from build123d import *

# Parameters (mm, degrees)
F1_DEPTH = 10
F3_DEPTH = 4.4
F4_R     = 7.5
F5_DEPTH = 3
F6_R     = 3
F7_DEPTH = 13.001


with BuildPart() as f1:
    # F0 (on Top) → F1 (new body)
    with BuildSketch(Plane.XY):
        with BuildLine():
            ThreePointArc((5.928073, 14.86129), (0, 19.582365), (-5.928073, 14.86129))
            ThreePointArc((-5.928073, 14.86129), (-6.94214, 14.415502), (-7.922931, 13.900617))
            ThreePointArc((-7.922931, 13.900617), (-15.31011, 12.209405), (-15.315118, 4.631108))
            ThreePointArc((-15.315118, 4.631108), (-15.598847, 3.560335), (-15.807807, 2.472496))
            ThreePointArc((-15.807807, 2.472496), (-19.091394, -4.357486), (-13.169566, -9.086392))
            ThreePointArc((-13.169566, -9.086392), (-12.509304, -9.975837), (-11.789082, -10.817465))
            ThreePointArc((-11.789082, -10.817465), (-8.49647, -17.643101), (-1.107063, -15.961654))
            ThreePointArc((-1.107063, -15.961654), (0, -16), (1.107063, -15.961654))
            ThreePointArc((1.107063, -15.961654), (8.49647, -17.643101), (11.789082, -10.817465))
            ThreePointArc((11.789082, -10.817465), (12.509304, -9.975837), (13.169566, -9.086392))
            ThreePointArc((13.169566, -9.086392), (19.091394, -4.357486), (15.807807, 2.472496))
            ThreePointArc((15.807807, 2.472496), (15.598847, 3.560335), (15.315118, 4.631108))
            ThreePointArc((15.315118, 4.631108), (15.31011, 12.209405), (7.922931, 13.900617))
            ThreePointArc((7.922931, 13.900617), (6.94214, 14.415502), (5.928073, 14.86129))
        make_face()
    extrude(amount=F1_DEPTH)

    # F2 (on face) → F3 (cut)
    with BuildSketch(Plane.XY.offset(10)):
        Polygon((2.875, -4.979646), (5.75, 0), (2.875, 4.979646), (-2.875, 4.979646), (-5.75, 0), (-2.875, -4.979646), align=None)
    extrude(amount=-F3_DEPTH, mode=Mode.SUBTRACT)

    # F4 (on face) → F5 (join)
    with BuildSketch(Plane(origin=(0, 0, 0), x_dir=(1, 0, 0), z_dir=(0, 0, -1))):
        Circle(F4_R)
    extrude(amount=F5_DEPTH)

    # F6 (on face) → F7 (cut, through all)
    with BuildSketch(Plane(origin=(0, 0, -3), x_dir=(1, 0, 0), z_dir=(0, 0, -1))):
        Circle(F6_R)
    extrude(amount=-F7_DEPTH, mode=Mode.SUBTRACT)


solid = f1.part
Work out the finished part from the listing and answer in its coordinate system (mm). A direction names the side the tool comes from. Give positions to 0.01 mm unless a question says otherwise; leave off trailing zeros. Loops run counter-clockwise (first coordinate to the right, second up) from the corner with the lowest first, then second, coordinate; pieces in that order, holes last. Notation, with made-up numbers: (80, 37) - (117, 37) arc R17 cw to (117, 44) - close; hole circle Ø1 at (50.5, 3.5). An arc over 180 degrees is marked (long way). Answer in a Markdown table with one row per item. Add a question column.
Q1. The part is cut by section C-C (y = 7). Determine the outline of the cut face in (x, z).
Q2. Determine the mould class of faces 4 (the cylindrical face through (0.11, 19.58, 4.93)), 5 (the flat face through (3.2, -0.1, -3)), 6 (the flat face through (4.333, 2.455, 7.831)) for opening direction Y: released by +Y, released by -Y, zero draft, split by the parting line, or undercut.
Q3. Consider line 1 along X through (y, z) = (0, -1); line 2 along Z through (x, y) = (-6, 12); line 3 along X through (y, z) = (0, 1.5). Determine where each line is inside the solid, lowest interval first.
Q4. The part is cut by section D-D (y = -4.5). Determine the outline of the cut face in (x, z), and give its area (3 significant figures).
Q5. Each of these flat-tipped pins is pushed along its axis until it touches: P1, Ø6, axis at y = -7.5, z = 4.5, coming from the +X side; P2, Ø3, axis at y = 3.5, z = 5, coming from the -X side; P3, Ø5, axis at x = 1, y = 2, coming from the +Z side. Where does it stop, or does it pass through?
Q6. The part is cut by section B-B (x = 0). Determine the outline of the cut face in (y, z), and give its area (3 significant figures).
Q7. A tool of negligible diameter and unlimited length cuts with its end or side. For faces 1 (the flat face through (-4.292, 2.525, 7.831)), 2 (the cylindrical face through (-15.595, 3.575, 4.93)), 3 (the flat face through (8, 1, 0)), from which of +Z, -Z, +X, -X, +Y, -Y can it reach the whole face along a straight path? Write none if from no direction.
Q8. The part is cut by section A-A (z = 4). Determine the outline of the cut face in (x, y).
Solution:
| question | item | result |
|---|---|---|
| 1 | outline | (-16.47, 0) - (-2.69, 0) - (-2.69, -3) - (2.69, -3) - (2.69, 0) - (16.47, 0) - (16.47, 10) - (-16.47, 10) - close |
| 2 | face 4 | released by +Y |
| 2 | face 5 | zero draft |
| 2 | face 6 | undercut |
| 3 | line 1 | x = -7.5 to -3, 3 to 7.5 |
| 3 | line 2 | z = 0 to 10 |
| 3 | line 3 | x = -18.45 to -3, 3 to 18.45 |
| 4 | outline | (-19.06, 0) - (-6, 0) - (-6, -3) - (6, -3) - (6, 0) - (19.06, 0) - (19.06, 10) - (3.15, 10) - (3.15, 5.6) - (-3.15, 5.6) - (-3.15, 10) - (-19.06, 10) - close |
| 4 | area | 389 mm² |
| 5 | P1 | stops at x = 19.06 |
| 5 | P2 | stops at x = -16.62 |
| 5 | P3 | stops at z = 5.6 |
| 6 | outline | (-16, 0) - (-7.5, 0) - (-7.5, -3) - (-3, -3) - (-3, 5.6) - (-4.98, 5.6) - (-4.98, 10) - (-16, 10) - close; (3, -3) - (7.5, -3) - (7.5, 0) - (19.58, 0) - (19.58, 10) - (4.98, 10) - (4.98, 5.6) - (3, 5.6) - close |
| 6 | area | 305 mm² |
| 7 | face 1 | +Z |
| 7 | face 2 | +Z, -Z, -X |
| 7 | face 3 | -Z |
| 8 | outline | (-15.81, 2.47) arc R6.08 ccw to (-13.17, -9.09) arc R16 ccw to (-11.79, -10.82) arc R6.08 ccw to (-1.11, -15.96) arc R16 ccw to (1.11, -15.96) arc R6.08 ccw to (11.79, -10.82) arc R16 ccw to (13.17, -9.09) arc R6.08 ccw to (15.81, 2.47) arc R16 ccw to (15.32, 4.63) arc R6.08 ccw to (7.92, 13.9) arc R16 ccw to (5.93, 14.86) arc R6.08 ccw to (-5.93, 14.86) arc R16 ccw to (-7.92, 13.9) arc R6.08 ccw to (-15.32, 4.63) arc R16 ccw to start; hole circle Ø6 at (0, 0) |
